Job drawing, mm, ordinate dimensions from the low corner. One solid piece. A direction names the side the tool comes from. Give positions to 0.01 mm unless a question says otherwise; leave off trailing zeros. Order: outer loops, then holes, each group sorted by start corner. A loop starts at its lowest first (then second) coordinate and runs counter-clockwise, first axis right, second up.
Item 1: Band-saw the part on A-A on x = 50.5. Give the cut face in (y, z) (3 decimals).
Item 2: Flat gauge pins, fed straight in: P1, Ø3, axis at x = 9.5, z = 25, coming from the +Y side; P2, Ø1.5, axis at y = 23, z = 13.5, coming from the +X side; P3, Ø6.5, axis at x = 50.5, z = 5, coming from the -Y side (3 decimals); P4, Ø9, axis at x = 25, z = 21, coming from the +Y side (3 decimals). Where does each tip first touch, or does it go through?
Item 3: Band-saw the part on B-B on z = 31. Give the cut face in (x, y), plus the area to 3 significant figures.
Item 4: Band-saw the part on D-D on x = 31.5. Give the cut face in (y, z) (3 decimals), plus the area to 4 significant figures.
Item 5: Wall check: L1, parallel to Z at x = 9.5, y = 27.25; L2, parallel to Y at x = 5, z = 34; L3, parallel to X at y = 33.75, z = 5. Give the ranges that are in metal, low to high.
Item 6: Band-saw the part on C-C on z = 5. Give the cut face in (x, y) (3 decimals), plus the area to 3 significant figures.
Item 7: Which spindle directions (+Z, -Z, +X, -X, +Y, -Y) get a long thin tool onto all of the face, cutting with end or side? Do the marked faces 1, 2, 3, 4 and 5. Say none if no direction does.
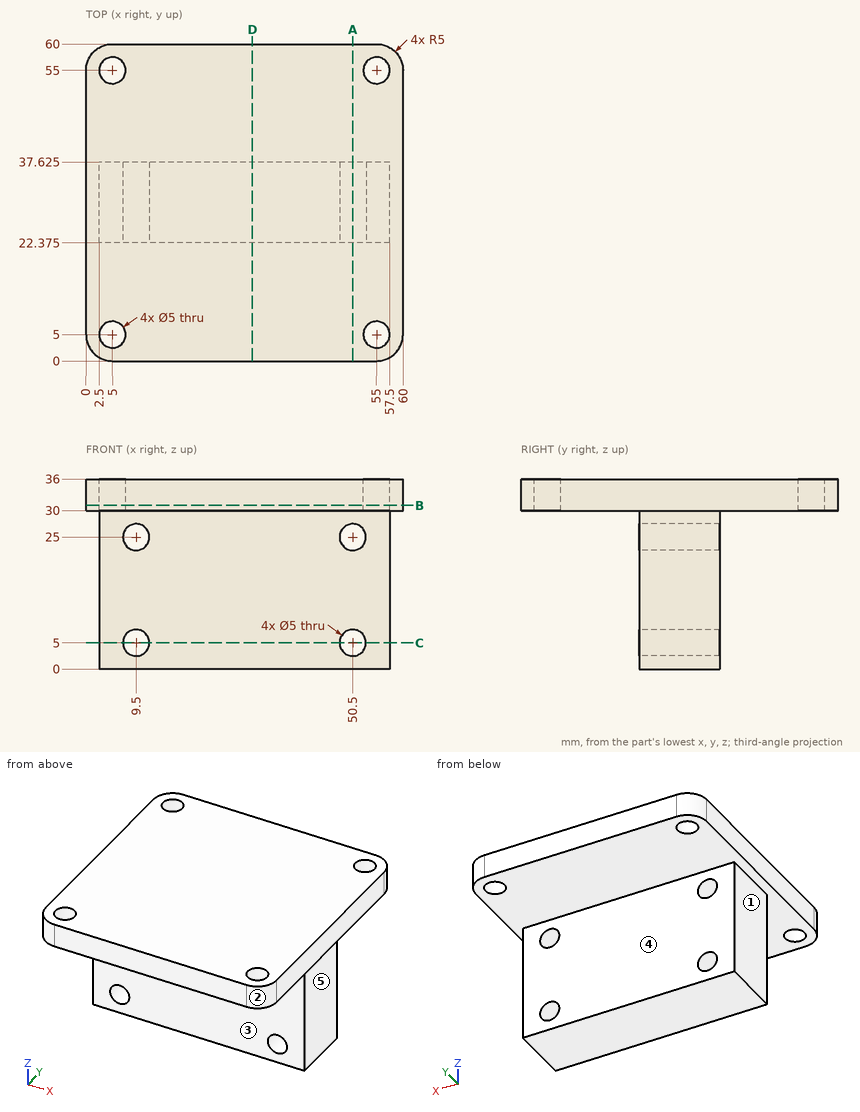
The answers:
1. outline: (0, 30) - (22.375, 30) - (22.375, 27.5) - (37.625, 27.5) - (37.625, 30) - (60, 30) - (60, 36) - (0, 36) - close; (22.375, 0) - (37.625, 0) - (37.625, 2.5) - (22.375, 2.5) - close; (22.375, 7.5) - (37.625, 7.5) - (37.625, 22.5) - (22.375, 22.5) - close
2. P1: passes through
2. P2: stops at x = 57.5
2. P3: stops at y = 22.375
2. P4: stops at y = 37.625
3. outline: (0, 5) arc R5 ccw to (5, 0) - (55, 0) arc R5 ccw to (60, 5) - (60, 55) arc R5 ccw to (55, 60) - (5, 60) arc R5 ccw to (0, 55) - close; hole circle Ø5 at (5, 5); hole circle Ø5 at (5, 55); hole circle Ø5 at (55, 5); hole circle Ø5 at (55, 55)
3. area: 3,500 mm2
4. outline: (0, 30) - (22.375, 30) - (22.375, 0) - (37.625, 0) - (37.625, 30) - (60, 30) - (60, 36) - (0, 36) - close
4. area: 817.5 mm2
5. L1: z = 0 to 2.5, 7.5 to 22.5, 27.5 to 36
5. L2: y = 0 to 2.5, 7.5 to 52.5, 57.5 to 60
5. L3: x = 2.5 to 7, 12 to 48, 53 to 57.5
6. outline: (2.5, 22.375) - (7, 22.375) - (7, 37.625) - (2.5, 37.625) - close; (12, 22.375) - (48, 22.375) - (48, 37.625) - (12, 37.625) - close; (53, 22.375) - (57.5, 22.375) - (57.5, 37.625) - (53, 37.625) - close
6. area: 686 mm2
7. face 1: -Z, -X, +Y, -Y
7. face 2: +Z, -Z, +X, -Y
7. face 3: -Z, +X, -X, -Y
7. face 4: -Z, +X, -X, +Y
7. face 5: -Z, +X, +Y, -Y
